from build123d import *

# Parameters (mm, degrees)
SKETCH1_W           = 220
SKETCH1_H           = 67
BOSS_EXTRUDE1_DEPTH = 2
SKETCH2_W           = 2
SKETCH2_H           = 33.5
CUT_EXTRUDE1_DEPTH  = 116.005434654


with BuildPart() as part:
    # Sketch1 → Boss-Extrude1 (new body)
    with BuildSketch(Plane.XY):
        Rectangle(SKETCH1_W, SKETCH1_H)
    extrude(amount=BOSS_EXTRUDE1_DEPTH)

    # Sketch2 → Cut-Extrude1 (cut, through all)
    with BuildSketch(Plane.XY.offset(2)):
        with Locations((-37, -16.75)):
            Rectangle(SKETCH2_W, SKETCH2_H)
        with Locations((-74, -16.75)):
            Rectangle(SKETCH2_W, SKETCH2_H)
        with Locations((74, -16.75)):
            Rectangle(SKETCH2_W, SKETCH2_H)
        with Locations((37, -16.75)):
            Rectangle(SKETCH2_W, SKETCH2_H)
        with Locations((0, -16.75)):
            Rectangle(SKETCH2_W, SKETCH2_H)
    extrude(amount=-CUT_EXTRUDE1_DEPTH, mode=Mode.SUBTRACT)


solid = part.part
For this review, take the finished solid that the model builds, in its own axes (mm). Round coordinates to 2 decimals unless told otherwise and drop trailing zeros. Order: outer loops, then holes, each group sorted by start corner. A loop starts at its lowest first (then second) coordinate and runs counter-clockwise, first axis right, second up. Notation, with made-up numbers: M -27,37 L -18,37 A23 ccw -18,65 Z; hole C 8.5,-24 d1. An arc over 180 degrees is marked long. Use a Markdown table: item, result. Add a question column.
Item 1: Add section B-B, the plane z = 1.4. Give the boundary of the cut face in (x, y).
Item 2: Add section A-A, the plane y = -16. Give the boundary of the cut face in (x, z).
Item 3: To check wall thickness, follow line 1 along X through (y, z) = (-26.5, 0.8); line 2 along Y through (x, z) = (0.5, 1.5). State the ranges of each line that lie inside material, in increasing order.
Item 4: Insertion check: pin 1 (1 mm diameter, centred on x = 37, z = 1.5, fed in from -Y). The pin has a flat end and moves straight along its axis. Give the tip position at first contact, or say it passes through.
Geometry results:
| question | item | result |
|---|---|---|
| 1 | outline | M -110,-33.5 L -75,-33.5 L -75,0 L -73,0 L -73,-33.5 L -38,-33.5 L -38,0 L -36,0 L -36,-33.5 L -1,-33.5 L -1,0 L 1,0 L 1,-33.5 L 36,-33.5 L 36,0 L 38,0 L 38,-33.5 L 73,-33.5 L 73,0 L 75,0 L 75,-33.5 L 110,-33.5 L 110,33.5 L -110,33.5 Z |
| 2 | outline | M -110,0 L -75,0 L -75,2 L -110,2 Z; M -73,0 L -38,0 L -38,2 L -73,2 Z; M -36,0 L -1,0 L -1,2 L -36,2 Z; M 1,0 L 36,0 L 36,2 L 1,2 Z; M 38,0 L 73,0 L 73,2 L 38,2 Z; M 75,0 L 110,0 L 110,2 L 75,2 Z |
| 3 | line 1 | x = -110 to -75, -73 to -38, -36 to -1, 1 to 36, 38 to 73, 75 to 110 |
| 3 | line 2 | y = 0 to 33.5 |
| 4 | pin 1 | stops at y = 0 |
